```python
from build123d import *

# Parameters (mm, degrees)
SKETCH1_W           = 75
SKETCH1_H           = 75
SKETCH1_R           = 1.5
SKETCH1_R_2         = 4.5
SKETCH1_R_3         = 4
BOSS_EXTRUDE1_DEPTH = 5
SKETCH3_W           = 16
SKETCH3_H           = 22
CUT_EXTRUDE1_DEPTH  = 5
FILLET1_R           = 8


with BuildPart() as part:
    # Sketch1 → Boss-Extrude1 (new body)
    with BuildSketch(Plane(origin=(0, 0, 0), x_dir=(-1, 0, 0), z_dir=(0, 0, 1))):
        Rectangle(SKETCH1_W, SKETCH1_H)
        with Locations(Location((9.5, 0, 0), (0, 0, 180))):
            Circle(SKETCH1_R, mode=Mode.SUBTRACT)
        with Locations(Location((-9.5, 0, 0), (0, 0, 180))):
            Circle(SKETCH1_R, mode=Mode.SUBTRACT)
        with Locations(Location((0, -8, 0), (0, 0, 180))):
            Circle(SKETCH1_R, mode=Mode.SUBTRACT)
        with Locations(Location((0, 8, 0), (0, 0, 180))):
            Circle(SKETCH1_R, mode=Mode.SUBTRACT)
        with Locations(Location((0, 0, 0), (0, 0, 180))):
            Circle(SKETCH1_R_2, mode=Mode.SUBTRACT)
        with Locations(Location((20.757359313, 29.242640687, 0), (0, 0, 180))):
            Circle(SKETCH1_R_3, mode=Mode.SUBTRACT)
        with Locations((29.242640687, 20.757359313)):
            Circle(SKETCH1_R_3, mode=Mode.SUBTRACT)
        with Locations((-29.242640687, -20.757359313)):
            Circle(SKETCH1_R_3, mode=Mode.SUBTRACT)
        with Locations(Location((-20.757359313, -29.242640687, 0), (0, 0, 180))):
            Circle(SKETCH1_R_3, mode=Mode.SUBTRACT)
        with Locations((20.757359313, -29.242640687)):
            Circle(SKETCH1_R_3, mode=Mode.SUBTRACT)
        with Locations(Location((29.242640687, -20.757359313, 0), (0, 0, 180))):
            Circle(SKETCH1_R_3, mode=Mode.SUBTRACT)
        with Locations((-20.757359313, 29.242640687)):
            Circle(SKETCH1_R_3, mode=Mode.SUBTRACT)
        with Locations(Location((-29.242640687, 20.757359313, 0), (0, 0, 180))):
            Circle(SKETCH1_R_3, mode=Mode.SUBTRACT)
    extrude(amount=BOSS_EXTRUDE1_DEPTH)

    # Sketch3 → Cut-Extrude1 (cut)
    with BuildSketch(Plane.XY.offset(5)):
        with Locations((0, 26.5)):
            Rectangle(SKETCH3_W, SKETCH3_H)
        with Locations((0, -26.5)):
            Rectangle(SKETCH3_W, SKETCH3_H)
    extrude(amount=-CUT_EXTRUDE1_DEPTH, mode=Mode.SUBTRACT)

    # Fillet1
    fillet1_edges = [part.edges().sort_by_distance(p)[0] for p in [
        (-37.5, -37.5, 2.5),
        (-8, -37.5, 2.5),
        (8, -15.5, 2.5),
        (-8, -15.5, 2.5),
        (8, -37.5, 2.5),
        (37.5, -37.5, 2.5),
        (37.5, 37.5, 2.5),
        (8, 37.5, 2.5),
        (8, 15.5, 2.5),
        (-8, 15.5, 2.5),
        (-8, 37.5, 2.5),
        (-37.5, 37.5, 2.5),
    ]]
    fillet(fillet1_edges, radius=FILLET1_R - 0.0001)  # a hair under: the kernel refuses the full size


solid = part.part
```
Could you check a few things on this model? Use its own coordinates, in mm. A direction names the side the tool comes from. Coordinates: 2 decimals unless noted, no trailing zeros. Order: outer loops, then holes, each group sorted by start corner. A loop starts at its lowest first (then second) coordinate and runs counter-clockwise, first axis right, second up. Notation, with made-up numbers: M 64,42 L 114,42 A37 ccw 114,81 Z; hole C 34,-23 d5. An arc over 180 degrees is marked long. Use a Markdown table: item, result. Add a question column.
Q1. Which directions (+Z, -Z, +X, -X, +Y, -Y) give clear straight access to the entire face, cutting with the end or side of a thin tool? Please do faces 1 (the cylindrical face through (-5.719, 17.906, 2.465)), 2 (the cylindrical face through (5.719, -17.906, 2.465)), 3 (the flat face through (-23, 37.5, 2)).
Q2. If I drill on L1, parallel to Y at x = -21, z = 1.25; L2, parallel to X at y = 30, z = 1.9 (3 decimals); L3, parallel to Y at x = -31.5, z = 0.9, over which ranges is the centre line in solid material (lowest first)?
Q3. I want a section at B-B on x = 9. List the corners of the cut face in (y, z) for me, then the cut area to 3 significant figures.
Q4. I want a section at A-A on y = -8. List the corners of the cut face in (x, z) for me, then the cut area to 3 significant figures.
Q5. I'm going to push a flat-ended pin straight in: pin 1 (7 mm diameter, centred on x = -20.76, y = -29.24, fed in from -Z). Where does the tip first touch, or does it pass through?
Q6. I want a section at D-D on x = -18.5. List the corners of the cut face in (y, z) for me.
Q7. I want a section at C-C on y = 0. List the corners of the cut face in (x, z) for me, then the cut area to 3 significant figures.
Q8. We'd pull the mould along X, two halves only. Please class faces 4 (the flat face through (-23, -37.5, 2)), 5 (the cylindrical face through (-20.237, 25.277, 2.465)), 6 (the cylindrical face through (35.219, 35.094, 2.535)), 7 (the cylindrical face through (-10.406, 35.219, 2.465)): pulls with the +X half, pulls with the -X half, needs draft (parallel to the pull), parting line crosses it, or undercut.
Checked values:
| question | item | result |
|---|---|---|
| 1 | face 1 | +Z, -Z, +Y |
| 1 | face 2 | +Z, -Z, -Y |
| 1 | face 3 | +Z, -Z, +X, -X, +Y |
| 2 | L1 | -37.5 to -33.24, -25.25 to 25.25, 33.24 to 37.5 |
| 2 | L2 | -37.484 to -24.685, -16.83 to -8.016, 8.016 to 16.83, 24.685 to 37.484 |
| 2 | L3 | -37.25 to -24.06, -17.46 to 17.46, 24.06 to 37.25 |
| 3 | outline | M -33.37,0 L -1.41,0 L -1.41,5 L -33.37,5 Z; M 1.41,0 L 33.37,0 L 33.37,5 L 1.41,5 Z |
| 3 | area | 320 mm² |
| 4 | outline | M -37.5,0 L -1.5,0 L -1.5,5 L -37.5,5 Z; M 1.5,0 L 37.5,0 L 37.5,5 L 1.5,5 Z |
| 4 | area | 360 mm² |
| 5 | pin 1 | through |
| 6 | outline | M -37.5,0 L -32.54,0 L -32.54,5 L -37.5,5 Z; M -25.94,0 L 25.94,0 L 25.94,5 L -25.94,5 Z; M 32.54,0 L 37.5,0 L 37.5,5 L 32.54,5 Z |
| 7 | outline | M -37.5,0 L -11,0 L -11,5 L -37.5,5 Z; M -8,0 L -4.5,0 L -4.5,5 L -8,5 Z; M 4.5,0 L 8,0 L 8,5 L 4.5,5 Z; M 11,0 L 37.5,0 L 37.5,5 L 11,5 Z |
| 7 | area | 300 mm² |
| 8 | face 4 | needs draft |
| 8 | face 5 | undercut |
| 8 | face 6 | pulls with the +X half |
| 8 | face 7 | undercut |
